Check sheet for the modelled part. Datum: model origin and axes. Units: mm. A direction names the side the tool comes from. Give positions to 0.01 mm unless a question says otherwise; leave off trailing zeros. Order: outer loops, then holes, each group sorted by start corner. A loop starts at its lowest first (then second) coordinate and runs counter-clockwise, first axis right, second up.
Autodesk Inventor part; units mm, degrees
ref_plane "YZ Plane" through (0, 0, 0) normal (1, 0, 0) x (0, 1, 0)
ref_plane "XZ Plane" through (0, 0, 0) normal (0, 1, 0) x (-1, 0, 0)
ref_plane "XY Plane" through (0, 0, 0) normal (0, 0, 1) x (1, 0, 0)
sketch "Sketch1" plane through (0, 0, 0) normal (0, 0, 1) x (1, 0, 0)
  line L0 (13.1171, -4.9434) -> (5.7797, -12.7707)
  line L1 (5.7797, -12.7707) -> (-4.9434, -13.1171)
  line L2 (-4.9434, -13.1171) -> (-12.7707, -5.7797)
  line L3 (-12.7707, -5.7797) -> (-13.1171, 4.9434)
  line L4 (-13.1171, 4.9434) -> (-5.7797, 12.7707)
  line L5 (-5.7797, 12.7707) -> (4.9434, 13.1171)
  line L6 (4.9434, 13.1171) -> (12.7707, 5.7797)
  line L7 (12.7707, 5.7797) -> (13.1171, -4.9434)
  point P0 (0, 0)
  point P1 (0, 0)
extrude "Extrusion1" add sketch "Sketch1" along normal blind 10
fillet "Fillet1" radius 2 15 edges at (-0.4182, 12.9439, 10) (4.9434, 13.1171, 5) (-5.7797, 12.7707, 5) (12.7707, 5.7797, 5) (8.857, 9.4484, 10) (13.1171, -4.9434, 5) (12.9439, 0.4182, 10) (5.7797, -12.7707, 5) (9.4484, -8.857, 10) (-4.9434, -13.1171, 5) (0.4182, -12.9439, 10) (-12.7707, -5.7797, 5) (-8.857, -9.4484, 10) (-12.9439, -0.4182, 10) (-9.4484, 8.857, 10)
sketch "Sketch2" plane through (0, 0, 0) normal (0, 0, -1) x (-1, 0, 0)
  circle A0 centre (0, 0) radius 16.569
extrude "Extrusion2" add sketch "Sketch2" along normal blind 2.6
fillet "Fillet2" radius 2 1 edges at (16.569, 0, -2.6)
sketch "Sketch3" plane through (0, 0, -2.6) normal (0, 0, -1) x (-1, 0, 0)
  circle A0 centre (0, 0) radius 8
  dimension "d7" = 16
extrude "Extrusion3" add sketch "Sketch3" along normal blind 34
thread "Thread1"
properties part number "AnnishNT"
(1) Cross-section at B-B on z = -11.5. Enter the section's corners in (x, y).
Response values:
outline: circle Ø16 at (0, 0)
(2) Cross-section at A-A on z = 1. Enter the section's corners in (x, y).
Response values:
outline: (-13.12, 4.94) - (-12.8, -4.95) arc R2 ccw to (-12.17, -6.35) - (-5.55, -12.55) arc R2 ccw to (-4.12, -13.09) - (4.95, -12.8) arc R2 ccw to (6.35, -12.17) - (12.55, -5.55) arc R2 ccw to (13.09, -4.12) - (12.8, 4.95) arc R2 ccw to (12.17, 6.35) - (5.55, 12.55) arc R2 ccw to (4.12, 13.09) - (-4.95, 12.8) arc R2 ccw to (-6.35, 12.17) - close
(3) Set-up check for faces 1 (the face through (5.702, -12.625, 4.056)), 2 (the face through (12.376, 0.336, 9.399)), 3 (the face through (-12.39, 0.08, 9.4)): record each of +Z, -Z, +X, -X, +Y, -Y from which the full face is reachable in a straight line by a thin tool's end or side.
Response values:
face 1: +Z, +X, -Y
face 2: +Z, +X, +Y
face 3: +Z, -X, -Y
(4) Gauge pin test, flat ends, axial feed: pin 1 Ø8 at (x, y) = (-11.5, 10) entering from -Z; pin 2 Ø12 at (x, z) = (0.5, -19.5) entering from -Y; pin 3 Ø10 at (y, z) = (-7.5, -25) entering from -X; pin 4 Ø1.5 at (x, z) = (9, -21) entering from +Y. Record the tip position at first contact, or that the pin passes through.
Response values:
pin 1: stops at z = -2.6
pin 2: stops at y = -8
pin 3: stops at x = -7.6
pin 4: passes through
(5) Material ranges on L1, parallel to Z at x = 6, y = -6; L2, parallel to X at y = 1, z = -10.5; L3, parallel to Y at x = 6, z = -23.5, recorded low to high.
Response values:
L1: z = -2.6 to 10
L2: x = -7.94 to 7.94
L3: y = -5.29 to 5.29
